Here's the drawing with two shaded views (mm, measured from the low corner). I have some questions. Coordinates: 2 decimals unless noted, no trailing zeros. Loops run counter-clockwise (first coordinate to the right, second up) from the corner with the lowest first, then second, coordinate; pieces in that order, holes last. Notation, with made-up numbers: (0.25, 53) -> (20.25, 53) arc R20 cw to (20.25, 86) -> close; hole circle Ø4 at (46, 78). An arc over 180 degrees is marked (long way). Answer as a JSON object with one key per item and string values. Group by question number.
Q1. I want a section at B-B on x = 4.29. Write out the boundary of the cut face in (y, z).
Q2. I want a section at C-C on y = 3.7. Write out the boundary of the cut face in (x, z).
Q3. I need wall thicknesses on line 1 (Z direction, x = 4.29, y = 2.4); line 2 (X direction, y = 3.9, z = 4.5) (1 decimal); line 3 (X direction, y = 3.1, z = 6.5). Which ranges of each line are inside material? Lowest first, please.
Q4. I want a section at A-A on z = 4.34. Write out the boundary of the cut face in (x, y), then the cut area to 3 significant figures.
Q5. Thinking about a two-plate mould opening in X: for the marked faces 1, 2, 3 and 4, which applies, released by +X, released by -X, zero draft, split by the parting line, or undercut?
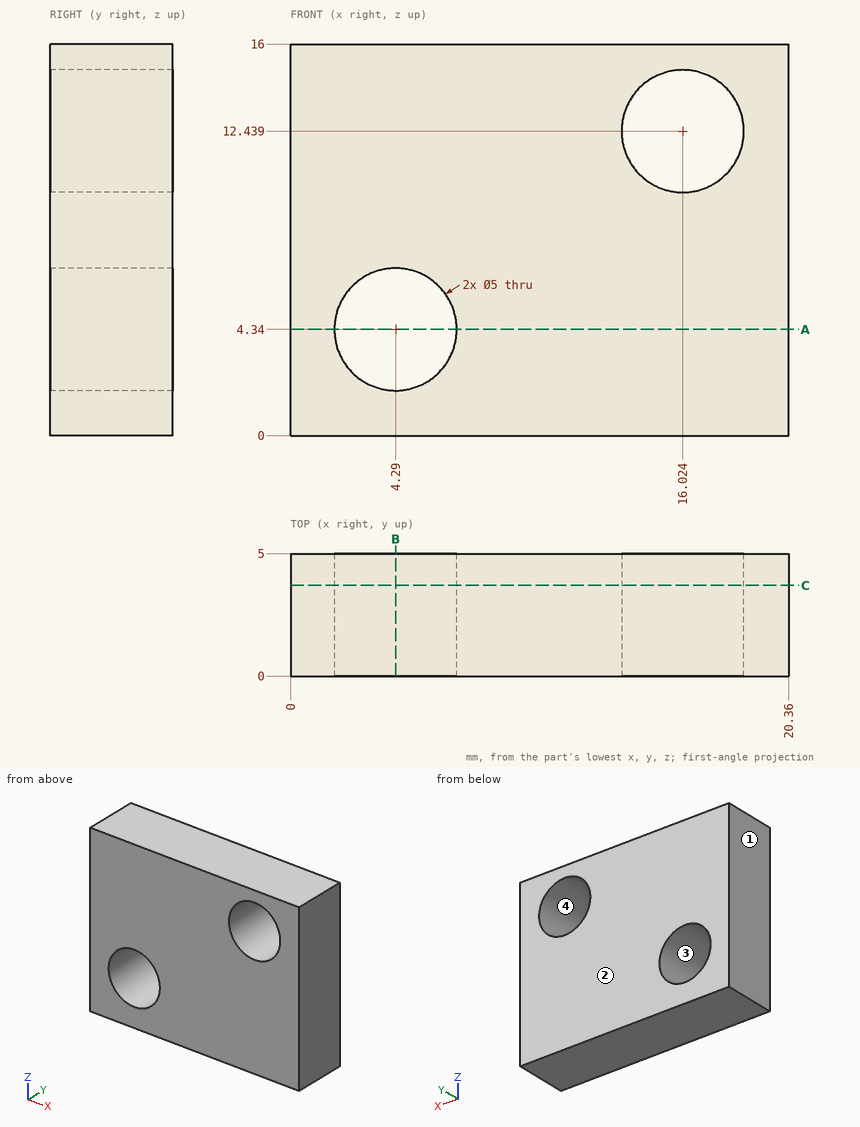
Result set:
{
 "1": {"outline": "(0, 0) -> (5, 0) -> (5, 1.84) -> (0, 1.84) -> close; (0, 6.84) -> (5, 6.84) -> (5, 16) -> (0, 16) -> close"},
 "2": {"outline": "(0, 0) -> (20.36, 0) -> (20.36, 16) -> (0, 16) -> close; hole circle Ø5 at (4.29, 4.34); hole circle Ø5 at (16.02, 12.44)"},
 "3": {"line 1": "z = 0 to 1.84, 6.84 to 16", "line 2": "x = 0 to 1.8, 6.8 to 20.4", "line 3": "x = 0 to 3.03, 5.55 to 20.36"},
 "4": {"outline": "(0, 0) -> (1.79, 0) -> (1.79, 5) -> (0, 5) -> close; (6.79, 0) -> (20.36, 0) -> (20.36, 5) -> (6.79, 5) -> close", "area": "76.8 mm²"},
 "5": {"face 1": "released by -X", "face 2": "zero draft", "face 3": "undercut", "face 4": "undercut"}
}
